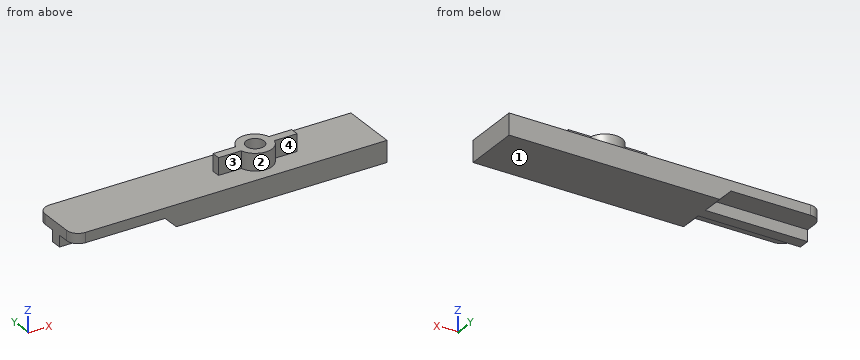
```python
from build123d import *

# Parameters (mm, degrees)
SKETCH_1_W          = 40
SKETCH_1_H          = 10
EXTRUDE_1_DEPTH     = 1.75
SKETCH_3_W          = 4
SKETCH_3_H          = 10
EXTRUDE_3_DEPTH     = 2
SKETCH_4_W          = 15
SKETCH_4_H          = 1.5
SKETCH_4_W_2        = 3
SKETCH_4_H_2        = 3.5
EXTRUDE_4_DEPTH     = 2
CHAMFER_1_SIZE      = 1
SKETCH_6_R          = 3
SKETCH_6_R_2        = 1.6
EXTRUDE_5_DEPTH     = 3
SKETCH_7_W          = 1.75
SKETCH_7_H          = 10
EXTRUDE_6_DEPTH     = 10
SKETCH_8_W          = 4
SKETCH_8_H          = 1.5
EXTRUDE_7_DEPTH     = 3
SKETCH_9_W          = 33
SKETCH_9_H          = 10
EXTRUDE_8_DEPTH     = 2
CHAMFER_2_SIZE      = 3
SKETCH_10_W         = 1.75
SKETCH_10_H         = 10
EXTRUDE_9_DEPTH     = 5
FILLET_1_R          = 2
CUT_EXTRUDE_START   = -1.75
SKETCH_11_R         = 1.6
CUT_EXTRUDE_1_DEPTH = 1.75
SKETCH_12_W         = 18
SKETCH_12_H         = 2
EXTRUDE_10_DEPTH    = 2


# Some blends are built 0.0001 mm under size
with BuildPart() as part:
    # 草图1 → 凸台-拉伸1 (new body)
    with BuildSketch(Plane.XY):
        with Locations((20, 5)):
            Rectangle(SKETCH_1_W, SKETCH_1_H)
    extrude(amount=EXTRUDE_1_DEPTH)

    # 草图3 → 凸台-拉伸3 (add)
    with BuildSketch(Plane(origin=(0, 0, 0), x_dir=(-1, 0, 0), z_dir=(0, 0, -1))):
        with Locations((-38, 5)):
            Rectangle(SKETCH_3_W, SKETCH_3_H)
    extrude(amount=EXTRUDE_3_DEPTH)

    # 草图4 → 凸台-拉伸4 (add)
    with BuildSketch(Plane(origin=(0, 0, 0), x_dir=(-1, 0, 0), z_dir=(0, 0, -1))):
        with Locations((-28.5, 5.75)):
            Rectangle(SKETCH_4_W, SKETCH_4_H)
        with Locations((-28.5, 4.25)):
            Rectangle(SKETCH_4_W, SKETCH_4_H)
        with Locations((-19.5, 5.75)):
            Rectangle(SKETCH_4_W_2, SKETCH_4_H)
        with Locations((-19.5, 4.25)):
            Rectangle(SKETCH_4_W_2, SKETCH_4_H)
        with Locations((-19.5, 8.25)):
            Rectangle(SKETCH_4_W_2, SKETCH_4_H_2)
        with Locations((-19.5, 1.75)):
            Rectangle(SKETCH_4_W_2, SKETCH_4_H_2)
        with Locations((-10.5, 5.75)):
            Rectangle(SKETCH_4_W, SKETCH_4_H)
        with Locations((-10.5, 4.25)):
            Rectangle(SKETCH_4_W, SKETCH_4_H)
        with Locations((-1.5, 5.75)):
            Rectangle(SKETCH_4_W_2, SKETCH_4_H)
        with Locations((-1.5, 4.25)):
            Rectangle(SKETCH_4_W_2, SKETCH_4_H)
        with Locations((-1.5, 8.25)):
            Rectangle(SKETCH_4_W_2, SKETCH_4_H_2)
        with Locations((-1.5, 1.75)):
            Rectangle(SKETCH_4_W_2, SKETCH_4_H_2)
    extrude(amount=EXTRUDE_4_DEPTH)

    # 倒角1
    chamfer_1_edges = [part.edges().sort_by_distance(p)[0] for p in [
        (10.5, 3.5, 0),
        (28.5, 3.5, 0),
    ]]
    chamfer(chamfer_1_edges, length=CHAMFER_1_SIZE)
    chamfer_1_2_edges = [part.edges().sort_by_distance(p)[0] for p in [
        (10.5, 3.5, -2),
        (28.5, 3.5, -2),
    ]]
    chamfer(chamfer_1_2_edges, length=CHAMFER_1_SIZE - 0.0001)  # a hair under: the kernel refuses the full size

    # 草图6 → 凸台-拉伸5 (add)
    with BuildSketch(Plane.XY.offset(1.75)):
        with Locations(Location((20, 5, 0), (0, 0, 180))):
            Circle(SKETCH_6_R)
        with Locations((20, 5)):
            Circle(SKETCH_6_R_2, mode=Mode.SUBTRACT)
    extrude(amount=EXTRUDE_5_DEPTH)

    # 草图7 → 凸台-拉伸6 (add)
    with BuildSketch(Plane.ZY):
        with Locations((0.875, 5)):
            Rectangle(SKETCH_7_W, SKETCH_7_H)
    extrude(amount=EXTRUDE_6_DEPTH)

    # 草图8 → 凸台-拉伸7 (add)
    with BuildSketch(Plane.XY.offset(1.75)):
        with Locations((15.09526249, 5)):
            Rectangle(SKETCH_8_W, SKETCH_8_H)
        with Locations((24.90473751, 5)):
            Rectangle(SKETCH_8_W, SKETCH_8_H)
    extrude(amount=EXTRUDE_7_DEPTH)

    # 草图9 → 凸台-拉伸8 (add)
    with BuildSketch(Plane(origin=(0, 0, 0), x_dir=(-1, 0, 0), z_dir=(0, 0, -1))):
        with Locations((-19.5, 5)):
            Rectangle(SKETCH_9_W, SKETCH_9_H)
    extrude(amount=EXTRUDE_8_DEPTH)

    # 倒角2
    # the kernel refuses this chamfer: 3 mm, written as the material it takes off along each edge
    with BuildSketch(Plane(origin=(0, -7.715048964, -2), x_dir=(0.9996219169112968, 0, -0.027495876610586348), z_dir=(0, 1, 0))) as chamfer_2_piece_1_section:
        Polygon((CHAMFER_2_SIZE * 0.999621916911, -CHAMFER_2_SIZE * 0.0274958766106), (-CHAMFER_2_SIZE * 0.0274958766106, -CHAMFER_2_SIZE * 0.999621916911), (0, 0), align=None)
    chamfer_2_piece_1 = extrude(amount=25.430097928, mode=Mode.PRIVATE)
    chamfer_2_piece_1 = split(chamfer_2_piece_1, bisect_by=Plane(origin=(1.092091005, 5, 0), z_dir=(0, 0, -1)), keep=Keep.TOP, mode=Mode.PRIVATE)
    add(chamfer_2_piece_1, mode=Mode.SUBTRACT)

    # 草图10 → 凸台-拉伸9 (add)
    with BuildSketch(Plane.ZY.offset(10)):
        with Locations((0.875, 5)):
            Rectangle(SKETCH_10_W, SKETCH_10_H)
    extrude(amount=EXTRUDE_9_DEPTH)

    # 圆角1
    fillet_1_edges = [part.edges().sort_by_distance(p)[0] for p in [
        (-15, 10, 0.875),
        (-15, 0, 0.875),
    ]]
    fillet(fillet_1_edges, radius=FILLET_1_R)

    # 草图11 → 切除-拉伸1 (cut)
    with BuildSketch(Plane.XY.offset(1.75).offset(CUT_EXTRUDE_START)):
        with Locations(Location((20, 5, 0), (0, 0, 180))):
            Circle(SKETCH_11_R)
    extrude(amount=CUT_EXTRUDE_1_DEPTH, mode=Mode.SUBTRACT)

    # 草图12 → 凸台-拉伸10 (add)
    with BuildSketch(Plane(origin=(0, 0, 0), x_dir=(-1, 0, 0), z_dir=(0, 0, -1))):
        with Locations((6, 5)):
            Rectangle(SKETCH_12_W, SKETCH_12_H)
    extrude(amount=EXTRUDE_10_DEPTH)


solid = part.part
```
The model under review builds one solid part; all positions refer to its coordinate system, in mm. Face numbers are marked on the shaded views. A direction names the side the tool comes from. Round coordinates to 2 decimals unless told otherwise and drop trailing zeros. Write each loop counter-clockwise with the first axis right and the second up, starting at its lowest first coordinate (ties: lowest second). Pieces come first, ordered by that corner, then holes. Notation, with made-up numbers: M -5,-13.5 L 22,-13.5 A13 ccw 22,-2.5 Z; hole C 58,39 d4. An arc over 180 degrees is marked long. Use CSV: the item, a comma, the result in double quotes. Start each with the question number.
(1) Tool access review of the marked faces 1, 2, 3 and 4: name each direction out of +Z, -Z, +X, -X, +Y, -Y from which nothing blocks a thin tool from reaching the whole face with its end or side.
(2) We need section A-A, the plane y = 5. State the section outline as (x, z) points, then the cut area to 3 significant figures.
(3) We need section B-B, the plane z = 3. State the section outline as (x, y) points, then the cut area to 3 significant figures.
(4) We need section C-C, the plane x = -7.5. State the section outline as (y, z) points, then the cut area to 3 significant figures.
(5) Clearance check with flat-ended pins moving along their axes: P1, Ø5, axis at x = -5.5, y = 9, coming from the +Z side; P2, Ø0.6, axis at x = -5.5, z = -1, coming from the -Y side; P3, Ø1.2, axis at y = 5, z = 3.5, coming from the -X side. State where each tip first meets the part, or that it passes through.
(6) For line 1 along X through (y, z) = (5, 3.75); line 2 along X through (y, z) = (5, 0.8); line 3 along Y through (x, z) = (20, 1.1), list the stretches that pass through material, from the lowest coordinate up.
(7) We need section D-D, the plane x = 20. State the section outline as (y, z) points.
Findings:
1,face 1,"-Z, +X, -X, +Y, -Y"
1,face 2,"+Z, -Y"
1,face 3,"+Z, -X, -Y"
1,face 4,"+Z, +X, -Y"
2,outline,"M -15,-2 L 40,-2 L 40,1.75 L 26.9,1.75 L 26.9,4.75 L 21.6,4.75 L 21.6,0 L 18.4,0 L 18.4,4.75 L 13.1,4.75 L 13.1,1.75 L -15,1.75 Z"
2,area,"232 mm^2"
3,outline,"M 13.1,4.25 L 17.1,4.25 A3 ccw 22.9,4.25 L 26.9,4.25 L 26.9,5.75 L 22.9,5.75 A3 ccw 17.1,5.75 L 13.1,5.75 Z; hole C 20,5 d3.2"
3,area,"32.0 mm^2"
4,outline,"M 0,0 L 4,0 L 4,-2 L 6,-2 L 6,0 L 10,0 L 10,1.75 L 0,1.75 Z"
4,area,"21.5 mm^2"
5,P1,"z = 1.75"
5,P2,"y = 4"
5,P3,"x = 13.1"
6,line 1,"13.1 to 18.4, 21.6 to 26.9"
6,line 2,"-15 to 18.4, 21.6 to 40"
6,line 3,"0 to 3.4, 6.6 to 10"
7,outline,"M 0,-2 L 10,-2 L 10,1.75 L 8,1.75 L 8,4.75 L 6.6,4.75 L 6.6,0 L 3.4,0 L 3.4,4.75 L 2,4.75 L 2,1.75 L 0,1.75 Z"
